```python
from build123d import *

# Parameters (mm, degrees)
BASE_FLANGE1_DEPTH      = 4.7752
EDGE_FLANGE1_DEPTH      = 50.8
EDGE_FLANGE1_BEND_DEPTH = 50.8
EDGE_FLANGE2_DEPTH      = 101.6
EDGE_FLANGE2_BEND_DEPTH = 101.6
SKETCH18_R              = 5.159375
SKETCH18_W              = 4.7625
SKETCH18_H              = 22.225
CUT_EXTRUDE1_DEPTH      = 158.639173972
SKETCH19_W              = 26.9875
SKETCH19_H              = 5.55625
CUT_EXTRUDE2_DEPTH      = 131.648559208
CUT_EXTRUDE3_DEPTH      = 131.648559208
CUT_EXTRUDE3_DEPTH_BACK = 131.648559208
SKETCH20_R              = 5.159375


# Sheet-metal steps are written as plain solids
with BuildPart() as part:
    # Sketch1 → Base-Flange1 (new body)
    with BuildSketch(Plane(origin=(0, 0, 0), x_dir=(1, 0, 0), z_dir=(0, 1, 0))):
        Polygon((49.2125, -28.575), (49.2125, 28.575), (50.8, 28.575), (50.8, 79.375), (-50.8, 79.375), (-50.8, -79.375), (50.8, -79.375), (50.8, -28.575), align=None)
    extrude(amount=-BASE_FLANGE1_DEPTH)

    # Edge-Flange1 section (across the edge) → Edge-Flange1 (add)
    with BuildSketch(Plane(origin=(56.7436, 0, -28.575), x_dir=(-1, 0, 0), z_dir=(0, 0, -1))):
        with BuildLine():
            Line((-4.7752, 5.9436), (-4.7752, 69.85))
            Line((-4.7752, 69.85), (0, 69.85))
            Line((0, 69.85), (0, 5.9436))
            ThreePointArc((0, 5.9436), (1.740840135, 1.740840135), (5.9436, 0))
            Line((5.9436, 0), (5.9436, -4.7752))
            ThreePointArc((5.9436, -4.7752), (-1.635736166, -1.635736166), (-4.7752, 5.9436))
        make_face()
    extrude(amount=EDGE_FLANGE1_DEPTH)

    # Edge-Flange1 section 2 (across the edge) → Edge-Flange1 bend (add)
    with BuildSketch(Plane(origin=(56.7436, 0, 79.375), x_dir=(-1, 0, 0), z_dir=(0, 0, -1))):
        with BuildLine():
            Line((-4.7752, 5.9436), (-4.7752, 69.85))
            Line((-4.7752, 69.85), (0, 69.85))
            Line((0, 69.85), (0, 5.9436))
            ThreePointArc((0, 5.9436), (1.740840135, 1.740840135), (5.9436, 0))
            Line((5.9436, 0), (5.9436, -4.7752))
            ThreePointArc((5.9436, -4.7752), (-1.635736166, -1.635736166), (-4.7752, 5.9436))
        make_face()
    extrude(amount=EDGE_FLANGE1_BEND_DEPTH)

    # Edge-Flange2 section (across the edge) → Edge-Flange2 (add)
    with BuildSketch(Plane(origin=(50.8, -4.7752, 86.9061), x_dir=(0, 0, -1), z_dir=(-1, 0, 0))):
        with BuildLine():
            Line((-4.7752, 5.9436), (-4.7752, 17.4498))
            Line((-4.7752, 17.4498), (0, 17.4498))
            Line((0, 17.4498), (0, 5.9436))
            ThreePointArc((0, 5.9436), (1.740840135, 1.740840135), (5.9436, 0))
            Line((5.9436, 0), (7.5311, 0))
            Line((7.5311, 0), (7.5311, -4.7752))
            Line((7.5311, -4.7752), (5.9436, -4.7752))
            ThreePointArc((5.9436, -4.7752), (-1.635736166, -1.635736166), (-4.7752, 5.9436))
        make_face()
    extrude(amount=EDGE_FLANGE2_DEPTH)

    # Edge-Flange2 section 2 (across the edge) → Edge-Flange2 bend (add)
    with BuildSketch(Plane(origin=(-50.8, -4.7752, -86.9061), x_dir=(0, 0, 1), z_dir=(1, 0, 0))):
        with BuildLine():
            Line((-4.7752, 5.9436), (-4.7752, 17.4498))
            Line((-4.7752, 17.4498), (0, 17.4498))
            Line((0, 17.4498), (0, 5.9436))
            ThreePointArc((0, 5.9436), (1.740840135, 1.740840135), (5.9436, 0))
            Line((5.9436, 0), (7.5311, 0))
            Line((7.5311, 0), (7.5311, -4.7752))
            Line((7.5311, -4.7752), (5.9436, -4.7752))
            ThreePointArc((5.9436, -4.7752), (-1.635736166, -1.635736166), (-4.7752, 5.9436))
        make_face()
    extrude(amount=EDGE_FLANGE2_BEND_DEPTH)

    # Sketch18 → Cut-Extrude1 (cut, symmetric)
    with BuildSketch(Plane.ZY.offset(-56.7436)):
        with Locations(Location((-53.975, 50.8, 0), (0, 0, 270))):
            Circle(SKETCH18_R)
        with Locations(Location((-53.975, 19.05, 0), (0, 0, 270))):
            Circle(SKETCH18_R)
        with Locations((-76.99375, 73.81875)):
            Rectangle(SKETCH18_W, SKETCH18_H)
        with Locations((-76.99375, 35.71875)):
            Rectangle(SKETCH18_W, SKETCH18_H)
    cut_extrude1 = extrude(amount=CUT_EXTRUDE1_DEPTH, both=True, mode=Mode.SUBTRACT)

    # Sketch19 → Cut-Extrude2 (cut, symmetric)
    with BuildSketch(Plane(origin=(0, 0, 0), x_dir=(1, 0, 0), z_dir=(0, 1, 0))):
        with Locations((-19.853275, 76.99375)):
            Rectangle(SKETCH19_W, SKETCH19_H)
        with Locations((18.246725, 76.99375)):
            Rectangle(SKETCH19_W, SKETCH19_H)
    cut_extrude2 = extrude(amount=CUT_EXTRUDE2_DEPTH, both=True, mode=Mode.SUBTRACT)

    # Sketch20 → Cut-Extrude3 (cut, two sides: drawn at the far end of the back side and taken through both)
    with BuildSketch(Plane(origin=(0, 0, 0), x_dir=(1, 0, 0), z_dir=(0, 1, 0)).offset(-CUT_EXTRUDE3_DEPTH_BACK)):
        with Locations((-101.437452915, 44.213567876)):
            Circle(SKETCH20_R)
        with Locations(Location((-31.75, 39.451067876, 0), (0, 0, 270))):
            Circle(SKETCH20_R)
        with Locations(Location((-38.677272727, -61.9125, 0), (0, 0, 270))):
            Circle(SKETCH20_R)
        with Locations((-108.364725642, -57.15)):
            Circle(SKETCH20_R)
    extrude(amount=CUT_EXTRUDE3_DEPTH + CUT_EXTRUDE3_DEPTH_BACK, mode=Mode.SUBTRACT)

    # Mirror1: Cut-Extrude1, Cut-Extrude2 across plane
    add(cut_extrude1.mirror(Plane.XY), mode=Mode.SUBTRACT)
    add(cut_extrude2.mirror(Plane.XY), mode=Mode.SUBTRACT)


solid = part.part
```
Can you work these out from the model? Positions are in its coordinate system, mm. A direction names the side the tool comes from. Give positions to 0.01 mm unless a question says otherwise; leave off trailing zeros. Loops run counter-clockwise (first coordinate to the right, second up) from the corner with the lowest first, then second, coordinate; pieces in that order, holes last. Notation, with made-up numbers: M -8,56 L 51,56 A16 ccw 51,65 Z; hole C -36,-4 d10. An arc over 180 degrees is marked long. Use CSV: the item, a comma, the result in double quotes. Start each with the question number.
1. If we mould it in two halves opening along X, with no side actions, what happens to faces 1 (the face through (-6.36, -2, 77)), 2 (the face through (58.296, -1.719, 54.331)), 3 (the face through (59, 62.706, -77))? For each: released by +X, released by -X, zero draft, split by the parting line, or undercut.
2. If I drill on L1, parallel to Z at x = 58, y = 19 (3 decimals); L2, parallel to Z at x = 26, y = -13; L3, parallel to Y at x = 42, z = -32.5, over which ranges is the centre line in solid material (lowest first)?
3. Imagine slicing it at B-B, the plane x = -9. Write out the boundary of the cut face in (y, z) (1 decimal), plus the area to 3 significant figures.
4. Imagine slicing it at D-D, the plane z = -62. Write out the boundary of the cut face in (x, y).
5. Imagine slicing it at C-C, the plane y = 50.8. Write out the boundary of the cut face in (x, z) (3 decimals).
6. Imagine slicing it at A-A, the plane y = -13. Write out the boundary of the cut face in (x, z), plus the area to 3 significant figures.
7. On a 3-axis mill with a long thin cutter (end or side, diameter ignored), from which of +Z, -Z, +X, -X, +Y, -Y can I reach the whole of each face in a straight line? I mean faces 4 (the face through (59, 62.706, 77)), 5 (the face through (-20, -2, 79.772)), 6 (the face through (49.212, -2, 0)). Say none if no direction works.
8. For P1, Ø4, axis at x = 60, y = 66.5, coming from the +Z side; P2, Ø2.5, axis at x = 59.5, z = 77.5, coming from the -Y side; P3, Ø5.5, axis at x = -20, y = -3, coming from the -Z side; P4, Ø10, axis at y = -10.5, z = -54, coming from the -X side, each with a flat end and sliding along its axis, tell me the tip position at first contact or that it passes through.
Response values:
1,face 1,"undercut"
1,face 2,"released by +X"
1,face 3,"zero draft"
2,L1,"-79.375 to -59.134, -48.816 to -28.575, 28.575 to 48.816, 59.134 to 79.375"
2,L2,"-91.68 to -86.91, 86.91 to 91.68"
2,L3,"-4.78 to 0"
3,outline,"M -22.2,-91.7 L -10.7,-91.7 A10.7 ccw 0,-81 L 0,-79.8 L -4.8,-79.8 L -4.8,-81 A5.9 cw -10.7,-86.9 L -22.2,-86.9 Z; M -22.2,86.9 L -10.7,86.9 A5.9 cw -4.8,81 L -4.8,79.8 L 0,79.8 L 0,81 A10.7 ccw -10.7,91.7 L -22.2,91.7 Z; M -4.8,-74.2 L 0,-74.2 L 0,74.2 L -4.8,74.2 Z"
3,area,"955 mm^2"
4,outline,"M -50.8,-4.78 L 50.8,-4.78 A10.72 ccw 61.52,5.94 L 61.52,69.85 L 56.74,69.85 L 56.74,5.94 A5.94 cw 50.8,0 L -50.8,0 Z"
5,outline,"M 56.744,-79.375 L 61.519,-79.375 L 61.519,-59.134 L 56.744,-59.134 Z; M 56.744,-48.816 L 61.519,-48.816 L 61.519,-28.575 L 56.744,-28.575 Z; M 56.744,28.575 L 61.519,28.575 L 61.519,48.816 L 56.744,48.816 Z; M 56.744,59.134 L 61.519,59.134 L 61.519,79.375 L 56.744,79.375 Z"
6,outline,"M -50.8,-91.68 L 50.8,-91.68 L 50.8,-86.91 L -50.8,-86.91 Z; M -50.8,86.91 L 50.8,86.91 L 50.8,91.68 L -50.8,91.68 Z"
6,area,"970 mm^2"
7,face 4,"+Z, +X, -X, +Y"
7,face 5,"+Y, -Y"
7,face 6,"+X, +Y, -Y"
8,P1,"z = 74.61"
8,P2,"y = -1.76"
8,P3,"z = -90.46"
8,P4,"through"
